```python
from build123d import *

# Parameters (mm, degrees)
SKETCH2_OUTSIDE_W           = 163.676
SKETCH2_OUTSIDE_H           = 163.676
SKETCH2_OUTSIDE_W_2         = 31.75
SKETCH2_OUTSIDE_H_2         = 36.068
CUT_EXTRUDE1_DEPTH          = 143.862884438
FILLET1_R                   = 1.27
FILLET2_R                   = 2.54
RINGCUT_EXTRUDE3_DEPTH      = 81.964552311
RINGCUT_EXTRUDE3_DEPTH_BACK = 81.964552311
SKETCH6_OUTSIDE_W           = 109.092
SKETCH6_OUTSIDE_H           = 109.092
SKETCH4_R                   = 1.9685
CUT_EXTRUDE2_DEPTH          = 71.484874378
RINGFILLET4_R               = 1.27
SKETCH7_R                   = 1.9685
CUT_EXTRUDE4_DEPTH          = 71.484874378


with BuildPart() as part:
    # Sketch1 → Revolve1 (revolve)
    with BuildSketch(Plane.XY, mode=Mode.PRIVATE) as revolve1_sk:
        Polygon((0, 0), (0.693363296, -1.905), (2.293363296, -1.905), (2.293363296, 2.4), (-34.231636704, 2.4), (-34.231636704, -60.325), (-31.056636704, -60.325), (-31.056636704, 0), (-13.69, 0), (-13.69, -3.2), (-12.09, -3.2), (-8.89, 0), align=None)
    revolve(revolve1_sk.sketch.rotate(Axis((-31.056636704, -60.325, 0), (-1, 0, 0)), 90), axis=Axis((-31.056636704, -60.325, 0), (-1, 0, 0)))

    # Sketch2 outside → Cut-Extrude1 (cut, through all)
    with BuildSketch(Plane(origin=(2.293363296, 0, 0), x_dir=(0, 0, -1), z_dir=(1, 0, 0))):
        with Locations((0, -60.325)):
            Rectangle(SKETCH2_OUTSIDE_W, SKETCH2_OUTSIDE_H)
        Rectangle(SKETCH2_OUTSIDE_W_2, SKETCH2_OUTSIDE_H_2, mode=Mode.SUBTRACT)
    extrude(amount=-CUT_EXTRUDE1_DEPTH, mode=Mode.SUBTRACT)

    # Fillet1
    fillet1_edges = [part.edges().sort_by_distance(p)[0] for p in [
        (-31.056636704, 0, 0),
    ]]
    fillet(fillet1_edges, radius=FILLET1_R)

    # Fillet2
    fillet2_edges = [part.edges().sort_by_distance(p)[0] for p in [
        (-34.231636704, 2.4, 0),
    ]]
    fillet(fillet2_edges, radius=FILLET2_R)

    # Sketch5 → RingRevolve2 (revolve)
    with BuildSketch(Plane.XY, mode=Mode.PRIVATE) as ringrevolve2_sk:
        Polygon((-31.056636704, -3.443742982), (-31.056636704, 10.02), (3.563363296, 10.02), (3.563363296, 23.241), (1.163363296, 23.241), (1.163363296, 12.42), (-31.056636704, 12.42), (-31.056636704, 23.241), (-34.231636704, 23.241), (-34.231636704, 11.15), (-34.231636704, -3.443742982), align=None)
    revolve(ringrevolve2_sk.sketch.rotate(Axis((-34.231636704, -18.034, 0), (1, 0, 0)), 90), axis=Axis((-34.231636704, -18.034, 0), (1, 0, 0)))

    # Sketch6 outside → RingCut-Extrude3 (cut, two sides: drawn at the far end of the back side and taken through both)
    with BuildSketch(Plane(origin=(2.293363296, 0, 0), x_dir=(0, 0, -1), z_dir=(1, 0, 0)).offset(-RINGCUT_EXTRUDE3_DEPTH_BACK)):
        with Locations((0, -18.034)):
            Rectangle(SKETCH6_OUTSIDE_W, SKETCH6_OUTSIDE_H)
        Polygon((-15.875, 0.357864138), (-15.875, -18.034), (15.875, -18.034), (15.875, 0.357864138), (15.875, 24.013762752), (-15.875, 24.013762752), align=None, mode=Mode.SUBTRACT)
    extrude(amount=RINGCUT_EXTRUDE3_DEPTH + RINGCUT_EXTRUDE3_DEPTH_BACK, mode=Mode.SUBTRACT)

    # Mirror1: part across plane


with BuildPart() as part_1:
    add(part.part)
    add(part.part.mirror(Plane(origin=(-34.231636704, -18.034, 15.875), x_dir=(0, 0, 1), z_dir=(0, -1, 0))))

    # Sketch4 → Cut-Extrude2 (cut, through all)
    with BuildSketch(Plane(origin=(-31.056636704, 0, 0), x_dir=(0, 0, -1), z_dir=(1, 0, 0))):
        with Locations((-9.525, -18.034)):
            Circle(SKETCH4_R)
        with Locations((9.525, -18.034)):
            Circle(SKETCH4_R)
    extrude(amount=-CUT_EXTRUDE2_DEPTH, mode=Mode.SUBTRACT)

    # RingFillet4
    ringfillet4_edges = [part_1.edges().sort_by_distance(p)[0] for p in [
        (-31.056636704, -38.468, 0),
        (-31.056636704, -46.088, 0),
        (1.163363296, -48.488, 0),
        (-31.056636704, -48.488, 0),
        (-31.056636704, 2.4, 0),
        (-31.056636704, 10.02, 0),
        (1.163363296, 12.42, 0),
        (-31.056636704, 12.42, 0),
    ]]
    fillet(ringfillet4_edges, radius=RINGFILLET4_R)

    # Sketch7 → Cut-Extrude4 (cut, through all)
    with BuildSketch(Plane(origin=(-31.056636704, 0, 0), x_dir=(0, 0, -1), z_dir=(1, 0, 0))):
        with Locations((0, 16.891)):
            Circle(SKETCH7_R)
        with Locations((0, -52.959)):
            Circle(SKETCH7_R)
    extrude(amount=-CUT_EXTRUDE4_DEPTH, mode=Mode.SUBTRACT)


solid = part_1.part
```
Geometry: final body of the model. Coordinates: model frame, mm. A direction names the side the tool comes from. Give positions to 0.01 mm unless a question says otherwise; leave off trailing zeros. Order: outer loops, then holes, each group sorted by start corner. A loop starts at its lowest first (then second) coordinate and runs counter-clockwise, first axis right, second up. Notation, with made-up numbers: M -25.5,57.25 L 27.5,57.25 A17 cw 27.5,75.25 Z; hole C 82.5,43.5 d2. An arc over 180 degrees is marked long. Answer as CSV lines item,"result". Start each with the question number.
1) Cut plane B-B (z = 0). State how many separate pieces and enclosed holes the cut face has, then the cut area to 3 significant figures.
2) Set-up query: faces 5 (the flat face through (2.293, 0, 0)), 6 (the cylindrical face through (-12.879, -32.868, 0.225)), 7 (the cylindrical face through (-32.622, -51.007, 0.256)). Return all of +Z, -Z, +X, -X, +Y, -Y with unobstructed straight access to the full face (end or side cutting, diameter ignored); none if empty.
3) Mould query, pull axis X, two halves, no side actions, for faces 1 (the cylindrical face through (-4.383, -36.068, 0.225)), 2 (the flat face through (-34.232, -17, 0)), 3 (the flat face through (-32, -19, -15.875)), 4 (the flat face through (2.293, -36, 0)). Classes: +X half, -X half, draft (parallel to the pull), parting line (faces both ways), or undercut.
4) First-contact query: P1, Ø5, axis at x = -13, z = 10, coming from the -Y side; P2, Ø1, axis at y = -37.5, z = -6, coming from the +X side; P3, Ø12, axis at x = -26.5, z = -11.5, coming from the -Y side. Flat tips, straight axial feed; report the tip coordinate or a pass-through.
5) Line query: line 1 (Y direction, x = -10, z = -0.5); line 2 (X direction, y = -53.5, z = 4.5); line 3 (Y direction, x = -22.5, z = 7.5). Output: solid intervals per line, ascending. Write a range as from..to.
6) Cut plane A-A (x = -25.5). Output: boundary loops of the cut face in (y, z) (3 decimals), then the cut area to 3 significant figures.
Findings below:
1,separate pieces,"3"
1,enclosed holes,"0"
1,area,"647 mm²"
2,face 5,"+Z, -Z, +X"
2,face 6,"+X"
2,face 7,"-X"
3,face 1,"undercut"
3,face 2,"-X half"
3,face 3,"draft"
3,face 4,"+X half"
4,P1,"stops at y = -47.55"
4,P2,"stops at x = 2.29"
4,P3,"stops at y = -58.6"
5,line 1,"y = -48.48..-46.08, -38.47..-34.96, -1.11..2.4, 10.02..12.42"
5,line 2,"x = -34.23..-31.06, 1.16..3.56"
5,line 3,"y = -47.55..-45.07, -38.02..-35.6, -0.47..1.95, 9..11.48"
6,outline,"M -44.023,-15.875 L -41.164,-15.875 A28.054 cw -41.164,15.875 L -44.023,15.875 A30.454 ccw Z; M -36.426,-15.875 L -33.942,-15.875 A60.325 cw -33.942,15.875 L -36.426,15.875 A62.725 ccw Z; M -2.126,-15.875 L 0.358,-15.875 A62.725 ccw 0.358,15.875 L -2.126,15.875 A60.325 cw Z; M 5.096,-15.875 L 7.955,-15.875 A30.454 ccw 7.955,15.875 L 5.096,15.875 A28.054 cw Z"
6,area,"315 mm²"
